```python
from build123d import *

# Parameters (mm, degrees)
F1_DEPTH      = 1000
F2_W          = 50
F2_H          = 200
F3_DEPTH      = 25
F3_DEPTH_BACK = 25
F4_W          = 175
F4_H          = 70
F5_DEPTH      = 25
F5_DEPTH_BACK = 25
F6_R          = 150
F7_R          = 100
F8_R          = 50


with BuildPart() as f1:
    # F0 (on Top) → F1 (new body)
    with BuildSketch(Plane.XY):
        Polygon((-25, 0), (-25, -25), (25, -25), (25, 25), (-25, 25), align=None)
    extrude(amount=F1_DEPTH)

    # F2 (on Front) → F3 (join, two sides)
    with BuildSketch(Plane.XZ) as f3_sk:
        Polygon((0, -50), (0, 0), (-150, 0), (-200, 0), (-200, -50), align=None)
        Polygon((150, 0), (0, 0), (0, -50), (200, -50), (200, 0), align=None)
        with Locations((-175, 100)):
            Rectangle(F2_W, F2_H)
        with Locations((175, 100)):
            Rectangle(F2_W, F2_H)
    extrude(amount=F3_DEPTH)
    extrude(f3_sk.sketch, amount=-F3_DEPTH_BACK)

    # F4 (on Front) → F5 (join, two sides)
    with BuildSketch(Plane.XZ) as f5_sk:
        with Locations((112.5, 235)):
            Rectangle(F4_W, F4_H)
        with Locations((-112.5, 235)):
            Rectangle(F4_W, F4_H)
    extrude(amount=F5_DEPTH)
    extrude(f5_sk.sketch, amount=-F5_DEPTH_BACK)

    # F6
    f6_edges = [f1.edges().sort_by_distance(p)[0] for p in [
        (200, 0, 270),
        (-200, 0, 270),
    ]]
    fillet(f6_edges, radius=F6_R)

    # F7
    f7_edges = [f1.edges().sort_by_distance(p)[0] for p in [
        (-200, 0, -50),
        (200, 0, -50),
    ]]
    fillet(f7_edges, radius=F7_R)

    # F8
    f8_edges = [f1.edges().sort_by_distance(p)[0] for p in [
        (-25, 0, 200),
        (25, 0, 200),
        (-150, 0, 200),
        (150, 0, 200),
        (-150, 0, 0),
        (150, 0, 0),
    ]]
    fillet(f8_edges, radius=F8_R)


solid = f1.part
```
Could you check a few things on this model? Use its own coordinates, in mm. A direction names the side the tool comes from. Give positions to 0.01 mm unless a question says otherwise; leave off trailing zeros. Order: outer loops, then holes, each group sorted by start corner. A loop starts at its lowest first (then second) coordinate and runs counter-clockwise, first axis right, second up.
Q1. For faces 1 (the flat face through (-200, 0, 85)), 2 (the flat face through (87, 0, 200)), 3 (the flat face through (37, 0, 270)), which set-ups out of +Z, -Z, +X, -X, +Y, -Y let a thin tool reach every point of the face, with its end or its side?
Q2. Suppose I cut it at B-B, the plane x = 131. Write out the boundary of the cut face in (y, z), and give its area (3 significant figures).
Q3. I'm going to push flat-ended pins straight in: P1, Ø4, axis at y = 12.5, z = 248.5, coming from the -X side; P2, Ø25, axis at x = 81, y = -9.5, coming from the +Z side; P3, Ø4, axis at x = 130, y = -13.5, coming from the +Z side. Where does each tip first touch, or does it pass through?
Q4. If I drill on line 1 along X through (y, z) = (10, 94.5); line 2 along X through (y, z) = (-15, 44); line 3 along X through (y, z) = (3.5, 427), over which ranges is the centre line in solid material (lowest first)?
Q5. We'd pull the mould along X, two halves only. Please class faces 4 (the flat face through (-16, 25, 283)), 5 (the flat face through (-25, 0, 630)), 6 (the cylindrical face through (40.036, 0.35, 185.742)): +X half, -X half, draft (parallel to the pull), parting line (faces both ways), or undercut.
Q6. Suppose I cut it at A-A, the plane y = 1. Write out the boundary of the cut face in (x, z).
Q7. Suppose I cut it at C-C, the plane z = 680.5. Write out the boundary of the cut face in (x, y).
Solution:
1. face 1: +Z, -Z, -X, +Y, -Y
1. face 2: +Y, -Y
1. face 3: +Z, +X, +Y, -Y
2. outline: (-25, -45.07) - (25, -45.07) - (25, 10.77) - (-25, 10.77) - close; (-25, 189.23) - (25, 189.23) - (25, 246.25) - (-25, 246.25) - close
2. area: 5,640 mm2
3. P1: stops at x = -130.61
3. P2: stops at z = 268.85
3. P3: stops at z = 248.12
4. line 1: x = -200 to -150, -25 to 25, 150 to 200
4. line 2: x = -199.82 to -149.64, -25 to 25, 149.64 to 199.82
4. line 3: x = -25 to 25
5. face 4: draft
5. face 5: -X half
5. face 6: undercut
6. outline: (-200, 50) arc R100 ccw to (-100, -50) - (100, -50) arc R100 ccw to (200, 50) - (200, 120) arc R150 ccw to (50, 270) - (25, 270) - (25, 1000) - (-25, 1000) - (-25, 270) - (-50, 270) arc R150 ccw to (-200, 120) - close; hole (-150, 50) arc R50 ccw to (-100, 0) - (-25, 0) - (-25, 150) arc R50 ccw to (-75, 200) - (-100, 200) arc R50 ccw to (-150, 150) - close; hole (25, 0) - (100, 0) arc R50 ccw to (150, 50) - (150, 150) arc R50 ccw to (100, 200) - (75, 200) arc R50 ccw to (25, 150) - close
7. outline: (-25, -25) - (25, -25) - (25, 25) - (-25, 25) - close
